```python
from build123d import *

# Parameters (mm, degrees)
MAIN_PLATE_DEPTH               = 3
BOTTOM_PLATE_CONNECTORS_DEPTH  = 22
REMOVE_STRESS_CONCENTRATIONS_R = 2.5
WIRE_HOLES_DEPTH               = 144.122325303
CUT_EXTRUDE1_DEPTH             = 144.614066163
FILLET1_R                      = 1.5


with BuildPart() as part:
    # Sketch1 → Main Plate (new body)
    with BuildSketch(Plane(origin=(0, 0, 0), x_dir=(1, 0, 0), z_dir=(0, 1, 0))):
        Polygon((-7, 100), (7, 100), (100, 7), (100, -7), (7, -100), (-7, -100), (-100, -7), (-100, 7), align=None)
    extrude(amount=MAIN_PLATE_DEPTH)

    # Sketch2 → Bottom Plate Connectors (add)
    with BuildSketch(Plane.XZ):
        Polygon((7.778174593, 16.970562748), (16.970562748, 7.778174593), (19.091883092, 9.899494937), (9.899494937, 19.091883092), align=None)
        Polygon((16.970562748, -7.778174593), (7.778174593, -16.970562748), (9.899494937, -19.091883092), (19.091883092, -9.899494937), align=None)
        Polygon((-7.778174593, -16.970562748), (-16.970562748, -7.778174593), (-19.091883092, -9.899494937), (-9.899494937, -19.091883092), align=None)
        Polygon((-16.970562748, 7.778174593), (-7.778174593, 16.970562748), (-9.899494937, 19.091883092), (-19.091883092, 9.899494937), align=None)
    extrude(amount=BOTTOM_PLATE_CONNECTORS_DEPTH)

    # Remove Stress Concentrations
    remove_stress_concentrations_edges = [part.edges().sort_by_distance(p)[0] for p in [
        (8.838834765, 0, 18.03122292),
        (18.03122292, 0, 8.838834765),
        (14.495689014, 0, 14.495689014),
        (18.03122292, 0, -8.838834765),
        (8.838834765, 0, -18.03122292),
        (14.495689014, 0, -14.495689014),
        (-8.838834765, 0, -18.03122292),
        (-18.03122292, 0, -8.838834765),
        (-14.495689014, 0, -14.495689014),
        (-18.03122292, 0, 8.838834765),
        (-8.838834765, 0, 18.03122292),
        (-14.495689014, 0, 14.495689014),
    ]]
    fillet(remove_stress_concentrations_edges, radius=REMOVE_STRESS_CONCENTRATIONS_R)

    # Sketch3 → Wire Holes (cut, through all)
    with BuildSketch(Plane.XZ):
        Polygon((30.405591591, -16.263455967), (38.890872965, -24.748737342), (24.748737342, -38.890872965), (16.263455967, -30.405591591), align=None)
        Polygon((-23.334523779, 30.405591591), (-19.798989873, 26.870057685), (-26.870057685, 19.798989873), (-30.405591591, 23.334523779), align=None)
    extrude(amount=-WIRE_HOLES_DEPTH, mode=Mode.SUBTRACT)

    # Sketch4 → Cut-Extrude1 (cut, through all)
    with BuildSketch(Plane(origin=(0, 3, 0), x_dir=(1, 0, 0), z_dir=(0, 1, 0))):
        Polygon((14.609127035, 85.319805153), (35.82233047, 64.106601718), (33.701010127, 61.985281374), (12.487806691, 83.19848481), align=None)
        Polygon((39.357864376, 60.571067812), (60.571067812, 39.357864376), (58.449747468, 37.236544033), (37.236544033, 58.449747468), align=None)
        Polygon((64.106601718, 35.82233047), (85.319805153, 14.609127035), (83.19848481, 12.487806691), (61.985281374, 33.701010127), align=None)
        Polygon((85.319805153, -14.609127035), (64.106601718, -35.82233047), (61.985281374, -33.701010127), (83.19848481, -12.487806691), align=None)
        Polygon((58.449747468, -37.236544033), (60.571067812, -39.357864376), (39.357864376, -60.571067812), (37.236544033, -58.449747468), align=None)
        Polygon((33.701010127, -61.985281374), (35.82233047, -64.106601718), (14.609127035, -85.319805153), (12.487806691, -83.19848481), align=None)
        Polygon((-14.609127035, -85.319805153), (-35.82233047, -64.106601718), (-33.701010127, -61.985281374), (-12.487806691, -83.19848481), align=None)
        Polygon((-37.236544033, -58.449747468), (-39.357864376, -60.571067812), (-60.571067812, -39.357864376), (-58.449747468, -37.236544033), align=None)
        Polygon((-61.985281374, -33.701010127), (-64.106601718, -35.82233047), (-85.319805153, -14.609127035), (-83.19848481, -12.487806691), align=None)
        Polygon((-85.319805153, 14.609127035), (-64.106601718, 35.82233047), (-61.985281374, 33.701010127), (-83.19848481, 12.487806691), align=None)
        Polygon((-58.449747468, 37.236544033), (-60.571067812, 39.357864376), (-39.357864376, 60.571067812), (-37.236544033, 58.449747468), align=None)
        Polygon((-33.701010127, 61.985281374), (-35.82233047, 64.106601718), (-14.609127035, 85.319805153), (-12.487806691, 83.19848481), align=None)
    extrude(amount=-CUT_EXTRUDE1_DEPTH, mode=Mode.SUBTRACT)

    # Fillet1
    fillet1_edges = [part.edges().sort_by_distance(p)[0] for p in [
        (16.263455967, 1.5, -30.405591591),
        (24.748737342, 1.5, -38.890872965),
        (30.405591591, 1.5, -16.263455967),
        (38.890872965, 1.5, -24.748737342),
        (-23.334523779, 1.5, 30.405591591),
        (-19.798989873, 1.5, 26.870057685),
        (-30.405591591, 1.5, 23.334523779),
        (-26.870057685, 1.5, 19.798989873),
        (-33.701010127, 1.5, 61.985281374),
        (-58.449747468, 1.5, 37.236544033),
        (-83.19848481, 1.5, 12.487806691),
        (-64.106601718, 1.5, -35.82233047),
        (-39.357864376, 1.5, -60.571067812),
        (-14.609127035, 1.5, -85.319805153),
        (14.609127035, 1.5, -85.319805153),
        (33.701010127, 1.5, 61.985281374),
        (58.449747468, 1.5, 37.236544033),
        (83.19848481, 1.5, 12.487806691),
        (39.357864376, 1.5, -60.571067812),
        (64.106601718, 1.5, -35.82233047),
        (-39.357864376, 1.5, 60.571067812),
        (-64.106601718, 1.5, 35.82233047),
        (-83.19848481, 1.5, -12.487806691),
        (-58.449747468, 1.5, -37.236544033),
        (-33.701010127, 1.5, -61.985281374),
        (33.701010127, 1.5, -61.985281374),
        (58.449747468, 1.5, -37.236544033),
        (83.19848481, 1.5, -12.487806691),
        (64.106601718, 1.5, 35.82233047),
        (-14.609127035, 1.5, 85.319805153),
        (39.357864376, 1.5, 60.571067812),
        (14.609127035, 1.5, 85.319805153),
        (-85.319805153, 1.5, 14.609127035),
        (-85.319805153, 1.5, -14.609127035),
        (-60.571067812, 1.5, -39.357864376),
        (-35.82233047, 1.5, -64.106601718),
        (-60.571067812, 1.5, 39.357864376),
        (-35.82233047, 1.5, 64.106601718),
        (12.487806691, 1.5, 83.19848481),
        (12.487806691, 1.5, -83.19848481),
        (-12.487806691, 1.5, 83.19848481),
        (-37.236544033, 1.5, 58.449747468),
        (-61.985281374, 1.5, 33.701010127),
        (-61.985281374, 1.5, -33.701010127),
        (-37.236544033, 1.5, -58.449747468),
        (-12.487806691, 1.5, -83.19848481),
        (35.82233047, 1.5, -64.106601718),
        (60.571067812, 1.5, -39.357864376),
        (85.319805153, 1.5, -14.609127035),
        (35.82233047, 1.5, 64.106601718),
        (60.571067812, 1.5, 39.357864376),
        (85.319805153, 1.5, 14.609127035),
        (37.236544033, 1.5, 58.449747468),
        (61.985281374, 1.5, 33.701010127),
        (37.236544033, 1.5, -58.449747468),
        (61.985281374, 1.5, -33.701010127),
    ]]
    fillet(fillet1_edges, radius=FILLET1_R - 0.0001)  # a hair under: the kernel refuses the full size


solid = part.part
```
The listing builds one solid part. Answer for the finished solid, in the listing's coordinates (mm). A direction names the side the tool comes from. Give positions to 0.01 mm unless a question says otherwise; leave off trailing zeros. Order: outer loops, then holes, each group sorted by start corner. A loop starts at its lowest first (then second) coordinate and runs counter-clockwise, first axis right, second up.
Item 1: The part is cut by section D-D, the plane z = 0. Give the vertices of the cut face in (x, y).
From the geometry:
outline: (-100, 0) - (100, 0) - (100, 3) - (-100, 3) - close
Item 2: The part is cut by section C-C, the plane x = 72.5. Give the vertices of the cut face in (y, z).
From the geometry:
outline: (0, -34.5) - (3, -34.5) - (3, -27.43) - (0, -27.43) - close; (0, -23.19) - (3, -23.19) - (3, 23.19) - (0, 23.19) - close; (0, 27.43) - (3, 27.43) - (3, 34.5) - (0, 34.5) - close
Item 3: Find the intervals of material crossed by probe 1 along Z at (x, y) = (18, 1); probe 2 along Y at (x, z) = (-75, 19.5); probe 3 along Z at (x, y) = (-63.5, 1), in increasing order.
From the geometry:
probe 1: z = -89 to -81.93, -77.69 to -32.14, -28.67 to 77.69, 81.93 to 89
probe 2: y = 0 to 3
probe 3: z = -43.5 to -35.07, -32.19 to 32.19, 35.07 to 43.5
Item 4: For a pull along X with two mould halves and no side action, classify faces 1 (the face through (25.35, 1.52, 74.58)), 2 (the face through (53, 1, -54)), 3 (the face through (13, -22, -13)) as pulls with the +X half, pulls with the -X half, needs draft (parallel to the pull), parting line crosses it, or undercut.
From the geometry:
face 1: undercut
face 2: pulls with the +X half
face 3: needs draft
Item 5: The part is cut by section B-B, the plane z = 43.5. Give the vertices of the cut face in (x, y), and give its area (3 significant figures).
From the geometry:
outline: (-63.5, 0) - (-56.43, 0) - (-56.43, 3) - (-63.5, 3) - close; (-52.19, 0) - (52.19, 0) - (52.19, 3) - (-52.19, 3) - close; (56.43, 0) - (63.5, 0) - (63.5, 3) - (56.43, 3) - close
area: 356 mm2
Item 6: Which of the six approach directions +Z, -Z, +X, -X, +Y, -Y give full straight-line access (tool end or side, diameter ignored) to faces 4 (the face through (54, 1, 53)), 5 (the face through (-12.46, -10.85, 12.29)), 6 (the face through (-22.961, 1.521, -72.726))?
From the geometry:
face 4: +Z, +X, +Y, -Y
face 5: -Y
face 6: +Y, -Y
Item 7: The part is cut by section A-A, the plane y = -19.25. Give the vertices of the cut face in (x, z), and give its area (3 significant figures).
From the geometry:
outline: (-19.09, -9.9) - (-9.9, -19.09) - (-7.78, -16.97) - (-16.97, -7.78) - close; (-19.09, 9.9) - (-16.97, 7.78) - (-7.78, 16.97) - (-9.9, 19.09) - close; (7.78, -16.97) - (9.9, -19.09) - (19.09, -9.9) - (16.97, -7.78) - close; (7.78, 16.97) - (16.97, 7.78) - (19.09, 9.9) - (9.9, 19.09) - close
area: 156 mm2
Item 8: Given pin 1 Ø10 at (x, z) = (40.5, 65.5) entering from -Y; pin 2 Ø1.5 at (x, y) = (-15, -9.5) entering from +Z; pin 3 Ø12 at (y, z) = (-15, -17) entering from +X, each flat-ended and moving along its own axis, determine where each tip first touches the part or whether it passes through.
From the geometry:
pin 1: stops at y = 0
pin 2: stops at z = 14.74
pin 3: stops at x = 17.99
